```python
from build123d import *

# Parameters (mm, degrees)
F1_DEPTH    = 25.4
F2_T        = -2.54
F3_T2_ANGLE = 222.0796162883
F3_T4_ANGLE = 132.0289295476
F3_T6_ANGLE = 132.0289295476
F5_DEPTH    = 2.54


# Not quite as in the source:
# - a fillet or chamfer that OpenCascade refuses, or shapes differently, is made with other operations: its cross-section is extruded or revolved along the edge and cut away or added


with BuildPart() as f1:
    # F0 (on Top) → F1 (new body)
    with BuildSketch(Plane.XY):
        with BuildLine():
            ThreePointArc((-27.94, 0), (-8.1834365336, -8.1834365336), (0, -27.94))
            ThreePointArc((0, -27.94), (8.1834365336, -8.1834365336), (27.94, 0))
            ThreePointArc((27.94, 0), (0, 27.94), (-27.94, 0))
        make_face()
    extrude(amount=F1_DEPTH)

    # F2
    f2_openings = [f1.faces().sort_by_distance(p)[0] for p in [
        (0, 7.974025, 25.4),
    ]]
    offset(amount=F2_T, openings=f2_openings)

    # F3: chamfer of 2.286 x 3.9594681461 on 3 edges, made by hand

    # F3_s1 → F3_t2 (revolve, cut)
    with BuildSketch(Plane(origin=(0, 0, 0), x_dir=(0, 0, 1), z_dir=(-0.359016499, -0.9333312132, 0))):
        Polygon((21.4405318539, -27.94), (25.4, -25.654), (25.4, -27.94), align=None)
    revolve(axis=Axis((0, 0, 25.4), (0, 0, 1)), revolution_arc=F3_T2_ANGLE, mode=Mode.SUBTRACT)

    # F3_s3 → F3_t4 (revolve, cut)
    with BuildSketch(Plane(origin=(-33.70000734, -12.9459832215, 0), x_dir=(0, 0, 1), z_dir=(-0.9334899239, -0.3586036279, 0))):
        Polygon((21.4405318539, 11.8776768894), (25.4, 14.1636768894), (25.4, 11.8776768894), align=None)
    revolve(axis=Axis((-27.94, -27.94, 25.4), (0, 0, -1)), revolution_arc=F3_T4_ANGLE, mode=Mode.SUBTRACT)

    # F3_s5 → F3_t6 (revolve, cut)
    with BuildSketch(Plane(origin=(12.9459832215, -33.70000734, 0), x_dir=(0, 0, 1), z_dir=(0.3586036279, -0.9334899239, 0))):
        Polygon((21.4405318539, 11.8776768894), (25.4, 14.1636768894), (25.4, 11.8776768894), align=None)
    revolve(axis=Axis((27.94, -27.94, 25.4), (0, 0, -1)), revolution_arc=F3_T6_ANGLE, mode=Mode.SUBTRACT)

    # F4 (on face) → F5 (cut, through all)
    with BuildSketch(Plane(origin=(0, 0, 0), x_dir=(1, 0, 0), z_dir=(0, 0, -1))):
        with BuildLine():
            ThreePointArc((-20.8487433266, -5.6087433266), (0, -21.59), (20.8487433266, -5.6087433266))
            ThreePointArc((20.8487433266, -5.6087433266), (9.138001762, -0.7355812889), (0, 8.06135568))
            ThreePointArc((0, 8.06135568), (-9.138001762, -0.7355812889), (-20.8487433266, -5.6087433266))
        make_face()
    extrude(amount=-F5_DEPTH, mode=Mode.SUBTRACT)


solid = f1.part
```
Here's how the part is built. I have some questions about the finished solid (model axes, mm). A direction names the side the tool comes from. Give positions to 0.01 mm unless a question says otherwise; leave off trailing zeros. Loops run counter-clockwise (first coordinate to the right, second up) from the corner with the lowest first, then second, coordinate; pieces in that order, holes last. Notation, with made-up numbers: M 43,50.5 L 91,50.5 A30 cw 91,89.5 Z; hole C 41.25,50.25 d8. An arc over 180 degrees is marked long. Put each result on its own line as item: value. Start each with the question number.
(1) If we mould it in two halves opening along Y, with no side actions, what happens to faces 1 (the conical face through (-11.8, -4.34, 22.57)), 2 (the cylindrical face through (0.614, 27.933, 10.57)), 3 (the cylindrical face through (-0.395, 21.586, 1.252))? For each: +Y half, -Y half, draft (parallel to the pull), parting line (faces both ways), or undercut.
(2) I need wall thicknesses on line 1 along X through (y, z) = (-4, 14.75); line 2 along Y through (x, z) = (-23, 16.5); line 3 along Y through (x, z) = (4.5, 4.75). Which ranges of each line are inside material? Lowest first, please. Write a range as [from, to].
(3) Will these pins go through, and if not, where does the flat tip stop? pin 1 Ø6 at (x, y) = (12, 15.5) entering from +Z; pin 2 Ø1 at (y, z) = (7.5, 10) entering from -X; pin 3 Ø3 at (x, z) = (-5, 22) entering from -Y.
(4) I want a section at B-B on z = 8. Please give me the cut outline in (x, y).
(5) For faces 4 (the cylindrical face through (0.525, 25.395, 13.81)), 5 (the cylindrical face through (7.97, -8.4, 10.57)), which set-ups out of +Z, -Z, +X, -X, +Y, -Y let a thin tool reach every point of the face, with its end or its side?
Answer block:
1. face 1: -Y half
1. face 2: +Y half
1. face 3: undercut
2. line 1: [-13.53, -9.07], [9.07, 13.53]
2. line 2: [-0.44, 2.14], [10.78, 15.86]
2. line 3: [-12.73, -8.46], [25, 27.58]
3. pin 1: z = 2.54
3. pin 2: x = -27.05
3. pin 3: y = -14.21
4. outline: M -27.94,0 A27.94 cw 0,-27.94 A27.94 cw 27.94,0 A27.94 ccw Z; hole M -25.28,2.42 A30.48 cw 0,-15.76 A30.48 cw 25.28,2.42 A25.4 ccw Z
5. face 4: +Z
5. face 5: +Z, -Z, +X, -Y
